from build123d import *

# Parameters (mm, degrees)
SKETCH_R           = 10.059441
PAD_DEPTH          = 10
SKETCH001_W        = 49.81546
SKETCH001_H        = 9.920586
PAD001_DEPTH       = 3
PAD002_DEPTH       = 7
SKETCH004_W        = 41.042639
SKETCH004_H        = 2.256016
PAD003_DEPTH       = 1
POLARPATTERN_COUNT = 5


with BuildPart() as part:
    # Sketch → Pad (new body)
    with BuildSketch(Plane.XY):
        Circle(SKETCH_R)
    extrude(amount=PAD_DEPTH)

    # Sketch001 (on Face3 of Pad) → Pad001 (join)
    with BuildSketch(Plane.XY.offset(10)):
        with Locations((24.90773, 4.960293)):
            Rectangle(SKETCH001_W, SKETCH001_H)
    pad001 = extrude(amount=-PAD001_DEPTH)

    # Sketch003 (on Face6 of Pad001) → Pad002 (join)
    with BuildSketch(Plane(origin=(0, 0, 7), x_dir=(1, 0, 0), z_dir=(0, 0, -1))):
        Polygon((49.81546, 0), (40.118187, 0), (40.118187, -7.363322), (0, -7.363322), (0, -9.920586), (49.81546, -9.920586), align=None)
    pad002 = extrude(amount=PAD002_DEPTH)

    # Sketch004 → Pad003 (join)
    with BuildSketch(Plane(origin=(0, 0, 7), x_dir=(1, 0, 0), z_dir=(0, 0, -1))):
        with Locations((22.09739, -1.128008)):
            Rectangle(SKETCH004_W, SKETCH004_H)
    pad003 = extrude(amount=PAD003_DEPTH)

    # PolarPattern: Pad001, Pad002, Pad003 ×5 about axis
    polarpattern_axis = Axis((0, 0, 10), (0, 0, 1))
    for i in range(1, POLARPATTERN_COUNT):
        add(pad001.rotate(polarpattern_axis, i * 360 / POLARPATTERN_COUNT))
        add(pad002.rotate(polarpattern_axis, i * 360 / POLARPATTERN_COUNT))
        add(pad003.rotate(polarpattern_axis, i * 360 / POLARPATTERN_COUNT))


solid = part.part
Here's how the part is built. I have some questions about the finished solid (model axes, mm). A direction names the side the tool comes from. Round coordinates to 2 decimals unless told otherwise and drop trailing zeros. Write each loop counter-clockwise with the first axis right and the second up, starting at its lowest first coordinate (ties: lowest second). Pieces come first, ordered by that corner, then holes.
1. I need wall thicknesses on L1, parallel to X at y = 1, z = 4.5; L2, parallel to X at y = 11, z = 6.25; L3, parallel to X at y = -22.5, z = 6.5. Which ranges of each line are inside material? Lowest first, please.
2. Suppose I cut it at A-A (x = -26). List the corners of the cut face in (y, z) for me, and give its area (3 significant figures).
3. For faces 5 (the flat face through (-21.348, 12.722, 6.507)), 6 (the flat face through (-43.26, 25.21, 5.07)), 7 (the flat face through (-28.13, -20.44, 7.29)), which set-ups out of +Z, -Z, +X, -X, +Y, -Y let a thin tool reach every point of the face, with its end or its side?
4. Will these pins go through, and if not, where does the flat tip stop? pin 1 Ø5 at (x, z) = (26.5, 7) entering from +Y; pin 2 Ø5 at (x, y) = (-21, -11.5) entering from +Z; pin 3 Ø6 at (x, y) = (-26, 17.5) entering from -Z; pin 4 Ø2 at (x, z) = (31, 2) entering from -Y.
5. If we mould it in two halves opening along Y, with no side actions, what happens to faces 1 (the flat face through (10.746, -33.073, 7.292)), 2 (the flat face through (-1.585, 27.226, 5.07)), 3 (the flat face through (49.815, 5, 5)), 4 (the flat face through (14.33, -20.28, 3.55))? For each: released by +Y, released by -Y, zero draft, split by the parting line, or undercut.
6. Suppose I cut it at C-C (y = 16). List the corners of the cut face in (x, z) for me, and give its area (3 significant figures).
7. Suppose I cut it at D-D (x = 26.5). List the corners of the cut face in (y, z) for me.
Answer sheet:
1. L1: x = -18.25 to -13.9, -10.01 to 10.11, 40.12 to 49.82
1. L2: x = -32.02 to -27.67, -18.98 to -15.14, -6.86 to -4.17, 1.2 to 3.57
1. L3: x = -30.97 to -27.13, -18.44 to -14.09, 7.31 to 9.68, 15.05 to 17.74
2. outline: (-31.15, 0) - (-27.99, 0) - (-27.99, 7) - (-21.68, 7) - (-21.68, 6) - (-18.89, 6) - (-18.89, 10) - (-31.15, 10) - close; (6.63, 0) - (9.79, 0) - (9.79, 7) - (16.1, 7) - (16.1, 6) - (18.89, 6) - (18.89, 10) - (6.63, 10) - close
2. area: 123 mm2
3. face 5: -Z
3. face 6: +Z, -Z, -X, +Y
3. face 7: +Z, -Z, -X
4. pin 1: stops at y = 9.92
4. pin 2: passes through
4. pin 3: stops at z = 6
4. pin 4: stops at y = 7.36
5. face 1: released by -Y
5. face 2: released by +Y
5. face 3: zero draft
5. face 4: undercut
6. outline: (-38.9, 0) - (-34.55, 0) - (-34.55, 7) - (-25.86, 7) - (-25.86, 6) - (-22.02, 6) - (-22.02, 10) - (-38.9, 10) - close; (-5.23, 0) - (-2.54, 0) - (-2.54, 7) - (2.83, 7) - (2.83, 6) - (5.2, 6) - (5.2, 10) - (-5.23, 10) - close
6. area: 137 mm2
7. outline: (0, 6) - (2.26, 6) - (2.26, 7) - (7.36, 7) - (7.36, 0) - (9.92, 0) - (9.92, 10) - (0, 10) - close
